from build123d import *

# Parameters (mm, degrees)
CUT_EXTRUDE1_DEPTH = 1.3
FILLET1_R          = 0.266
CHAMFER2_SIZE      = 0.3065


with BuildPart() as part:
    # Sketch1 → Revolve1 (revolve)
    with BuildSketch(Plane(origin=(0, 0, 0), x_dir=(-1, 0, 0), z_dir=(0, 0, -1)), mode=Mode.PRIVATE) as revolve1_sk:
        Polygon((0, 0), (2.86, 0), (2.86, 2.66), (0, 2.66), (0, 1.5), (-230, 1.5), (-230, 0), align=None)
    revolve(revolve1_sk.sketch.rotate(Axis((0, 0, 0), (-1, 0, 0)), 180), axis=Axis((0, 0, 0), (-1, 0, 0)))

    # Sketch2 → Cut-Extrude1 (cut)
    with BuildSketch(Plane.ZY.offset(2.86)):
        Polygon((-1.25, -0.721687836), (0, -1.443375673), (1.25, -0.721687836), (1.25, 0.721687836), (0, 1.443375673), (-1.25, 0.721687836), align=None)
    extrude(amount=-CUT_EXTRUDE1_DEPTH, mode=Mode.SUBTRACT)

    # Fillet1
    fillet1_edges = [part.edges().sort_by_distance(p)[0] for p in [
        (-2.86, 2.66, 0),
    ]]
    fillet(fillet1_edges, radius=FILLET1_R)

    # Chamfer2
    chamfer2_edges = [part.edges().sort_by_distance(p)[0] for p in [
        (230, 1.5, 0),
    ]]
    chamfer(chamfer2_edges, length=CHAMFER2_SIZE)


solid = part.part
For this review, take the finished solid that the model builds, in its own axes (mm). A direction names the side the tool comes from. Give positions to 0.01 mm unless a question says otherwise; leave off trailing zeros. Loops run counter-clockwise (first coordinate to the right, second up) from the corner with the lowest first, then second, coordinate; pieces in that order, holes last.
Item 1: Tool access review of faces 1 (the flat face through (0, 0, -2)), 2 (the cylindrical face through (-1.279, -2.537, 0.799)): name each direction out of +Z, -Z, +X, -X, +Y, -Y from which nothing blocks a thin tool from reaching the whole face with its end or side.
Item 2: For line 1 along X through (y, z) = (0.5, -1.7); line 2 along X through (y, z) = (1.05, -0.35); line 3 along Y through (x, z) = (18.5, -0.5), list the stretches that pass through material, from the lowest coordinate up.
Item 3: Take a section at A-A, the plane x = 148.5. State the section outline as (y, z) points, and give its area (3 significant figures).
Item 4: Insertion check: pin 1 (3 mm diameter, centred on y = 0.5, z = -1.5, fed in from +X); pin 2 (0.8 mm diameter, centred on y = 0, z = 0, fed in from -X); pin 3 (3 mm diameter, centred on x = 81, z = 2, fed in from -Y); pin 4 (2 mm diameter, centred on x = 50, y = -1.5, fed in from +Z). Each pin has a flat end and moves straight along its axis. Give the tip position at first contact, or say it passes through.
Calculated:
1. face 1: +X
1. face 2: +X, -X
2. line 1: x = -2.86 to 0
2. line 2: x = -1.56 to 230
2. line 3: y = -1.41 to 1.41
3. outline: circle Ø3 at (0, 0)
3. area: 7.07 mm2
4. pin 1: stops at x = 230
4. pin 2: stops at x = -1.56
4. pin 3: stops at y = -1.41
4. pin 4: stops at z = 1.41
